Study the drawing (mm; zero at the part's minimum x, y, z) and answer. Round coordinates to 2 decimals unless told otherwise and drop trailing zeros. Write each loop counter-clockwise with the first axis right and the second up, starting at its lowest first coordinate (ties: lowest second). Pieces come first, ordered by that corner, then holes.
(1) Each of these flat-tipped pins is pushed along its axis until it touches: pin 1 Ø1.9 at (x, y) = (35, 8) entering from +Z (3 decimals); pin 2 Ø8 at (x, z) = (9.5, 36.5) entering from -Y; pin 3 Ø1.9 at (x, y) = (37, 2) entering from +Z; pin 4 Ø1.1 at (y, z) = (3, 58.5) entering from -X. Where does it stop, or does it pass through?
(2) A cutting plane is placed at C-C, the plane x = 54.5. Give the vertices of the cut face in (y, z) (3 decimals), and give its area (3 significant figures).
(3) A cutting plane is placed at D-D, the plane x = 80.5. Give the vertices of the cut face in (y, z) (3 decimals), and give its area (3 significant figures).
(4) A cutting plane is placed at A-A, the plane z = 85.5. Give the vertices of the cut face in (x, y) (3 decimals).
(5) A cutting plane is placed at B-B, the plane y = 5.75. Give the vertices of the cut face in (x, z) (3 decimals), and give its area (3 significant figures).
(6) The mould has two halves that part along X. Classify the marked faces 1, 2 and 3: +X half, -X half, draft (parallel to the pull), parting line (faces both ways), or undercut.
(7) Find the intervals of material crossed by probe 1 along X at (y, z) = (6.5, 88) (3 decimals); probe 2 along X at (y, z) = (1.25, 82); probe 3 along Y at (x, z) = (11, 70.5), in increasing order.
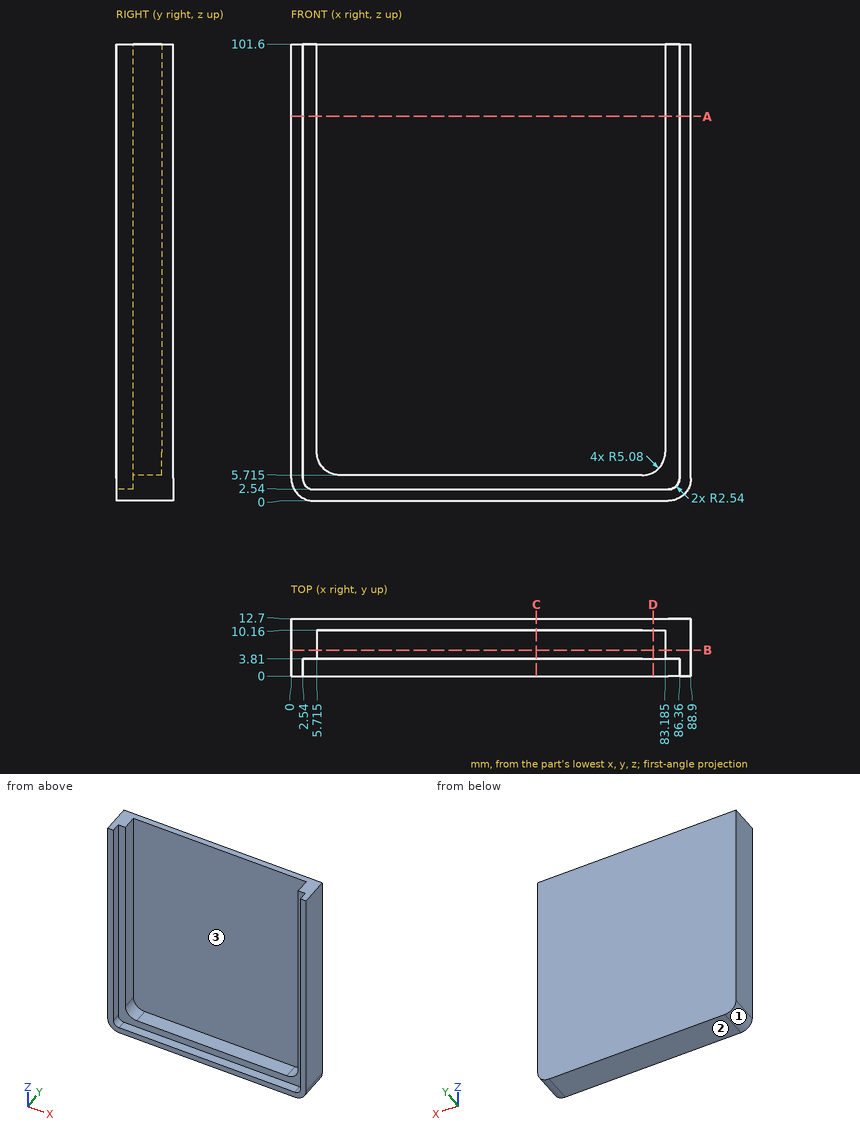
Solutions:
1. pin 1: stops at z = 5.715
1. pin 2: stops at y = 3.81
1. pin 3: stops at z = 2.54
1. pin 4: stops at x = 0
2. outline: (0, 0) - (12.7, 0) - (12.7, 101.6) - (10.16, 101.6) - (10.16, 5.715) - (3.81, 5.715) - (3.81, 2.54) - (0, 2.54) - close
2. area: 304 mm2
3. outline: (0, 0) - (12.7, 0) - (12.7, 101.6) - (10.16, 101.6) - (10.16, 6.315) - (3.81, 6.315) - (3.81, 2.54) - (0, 2.54) - close
3. area: 308 mm2
4. outline: (0, 0) - (2.54, 0) - (2.54, 3.81) - (5.715, 3.81) - (5.715, 10.16) - (83.185, 10.16) - (83.185, 3.81) - (86.36, 3.81) - (86.36, 0) - (88.9, 0) - (88.9, 12.7) - (0, 12.7) - close
5. outline: (0, 5.08) arc R5.08 ccw to (5.08, 0) - (83.82, 0) arc R5.08 ccw to (88.9, 5.08) - (88.9, 101.6) - (83.185, 101.6) - (83.185, 10.795) arc R5.08 cw to (78.105, 5.715) - (10.795, 5.715) arc R5.08 cw to (5.715, 10.795) - (5.715, 101.6) - (0, 101.6) - close
5. area: 1,600 mm2
6. face 1: -X half
6. face 2: draft
6. face 3: undercut
7. probe 1: x = 0 to 5.715, 83.185 to 88.9
7. probe 2: x = 0 to 2.54, 86.36 to 88.9
7. probe 3: y = 10.16 to 12.7
